from build123d import *

# Parameters (mm, degrees)
SKETCH1_W           = 45.3
SKETCH1_H           = 30
BOSS_EXTRUDE1_DEPTH = 7
SKETCH2_W           = 45.3
SKETCH2_H           = 24.294385672
CUT_EXTRUDE1_DEPTH  = 6
SKETCH5_W           = 12
SKETCH5_H           = 5.5
SKETCH5_W_2         = 10
SKETCH5_H_2         = 7
CUT_EXTRUDE2_DEPTH  = 7


with BuildPart() as part:
    # Sketch1 → Boss-Extrude1 (new body)
    with BuildSketch(Plane.XY):
        with Locations((5.590822785, 11.37721519)):
            Rectangle(SKETCH1_W, SKETCH1_H)
    extrude(amount=BOSS_EXTRUDE1_DEPTH)

    # Sketch2 → Cut-Extrude1 (cut)
    with BuildSketch(Plane.XY.offset(7)):
        with Locations((5.590822785, 8.524408026)):
            Rectangle(SKETCH2_W, SKETCH2_H)
    extrude(amount=-CUT_EXTRUDE1_DEPTH, mode=Mode.SUBTRACT)

    # Sketch5 → Cut-Extrude2 (cut)
    with BuildSketch(Plane(origin=(0, 26.37721519, 0), x_dir=(1, 0, 0), z_dir=(0, 1, 0))):
        with Locations((5.590822785, -2.75)):
            Rectangle(SKETCH5_W, SKETCH5_H)
        with Locations((-12.059177215, -3.5)):
            Rectangle(SKETCH5_W_2, SKETCH5_H_2)
        with Locations((23.240822785, -3.5)):
            Rectangle(SKETCH5_W_2, SKETCH5_H_2)
    extrude(amount=-CUT_EXTRUDE2_DEPTH, mode=Mode.SUBTRACT)


solid = part.part
Read the model definition and answer for the solid it produces. Units are mm, in the model's axes. A direction names the side the tool comes from. Give positions to 0.01 mm unless a question says otherwise; leave off trailing zeros. Write each loop counter-clockwise with the first axis right and the second up, starting at its lowest first coordinate (ties: lowest second). Pieces come first, ordered by that corner, then holes. Notation, with made-up numbers: (-23.5, 86.25) - (31.5, 86.25) arc R24 ccw to (31.5, 104.25) - close; hole circle Ø4 at (17, 47). An arc over 180 degrees is marked (long way). Return JSON: item names as keys, results as strings.
Q1. For faces 1 (the face through (5, 9, 1)), 2 (the face through (5.5, 19.377, 0.5)), 3 (the face through (18.241, 24, 4)), 4 (the face through (6, 24, 5.5)), 5 (the face through (-0.409, 24, 3)), determine the directions among +Z, -Z, +X, -X, +Y, -Y from which every point of the face is accessible in a straight line to the end or side of a thin tool.
Reply:
{"face 1": "+Z, +X, -X, -Y", "face 2": "+Z, -Z, +Y", "face 3": "+Z, -Z, +X, +Y", "face 4": "-Z, +Y, -Y", "face 5": "-Z, +Y"}
Q2. For a pull along X with two mould halves and no side action, classify faces 6 (the face through (11.591, 24, 3)), 7 (the face through (5, 20.672, 6)), 8 (the face through (28.241, 7.7, 0.5)) as released by +X, released by -X, zero draft, split by the parting line, or undercut.
Reply:
{"face 6": "undercut", "face 7": "zero draft", "face 8": "released by +X"}
Q3. Consider line 1 along Z through (x, y) = (2, -1.5); line 2 along X through (y, z) = (25, 3); line 3 along Y through (x, z) = (9.5, 6.75). Determine where each line is inside the solid, lowest interval first. Write a range as [from, to].
Reply:
{"line 1": "[0, 1]", "line 2": "[-7.06, -0.41], [11.59, 18.24]", "line 3": "[20.67, 26.38]"}
Q4. A cutting plane is placed at B-B, the plane x = 4. Determine the outline of the cut face in (y, z), and give its area (3 significant figures).
Reply:
{"outline": "(-3.62, 0) - (19.38, 0) - (19.38, 1) - (-3.62, 1) - close; (20.67, 5.5) - (26.38, 5.5) - (26.38, 7) - (20.67, 7) - close", "area": "31.6 mm²"}
Q5. A cutting plane is placed at A-A, the plane z = 1.75. Determine the outline of the cut face in (x, y), and give its area (3 significant figures).
Reply:
{"outline": "(-7.06, 20.67) - (-0.41, 20.67) - (-0.41, 26.38) - (-7.06, 26.38) - close; (11.59, 20.67) - (18.24, 20.67) - (18.24, 26.38) - (11.59, 26.38) - close", "area": "75.9 mm²"}
Q6. A cutting plane is placed at C-C, the plane x = -6. Determine the outline of the cut face in (y, z), and give its area (3 significant figures).
Reply:
{"outline": "(-3.62, 0) - (26.38, 0) - (26.38, 7) - (20.67, 7) - (20.67, 1) - (-3.62, 1) - close", "area": "64.2 mm²"}
Q7. Given P1, Ø2, axis at x = 18.5, y = 6.5, coming from the +Z side; P2, Ø0.5, axis at x = 23.5, z = 0.5, coming from the +Y side; P3, Ø1.6, axis at y = 23.5, z = 4, coming from the -X side, each flat-ended and moving along its own axis, determine where each tip first touches the part or whether it passes through.
Reply:
{"P1": "z = 1", "P2": "y = 19.38", "P3": "x = -7.06"}
Q8. A cutting plane is placed at D-D, the plane y = 9. Determine the outline of the cut face in (x, z), and give its area (3 significant figures).
Reply:
{"outline": "(-17.06, 0) - (28.24, 0) - (28.24, 1) - (-17.06, 1) - close", "area": "45.3 mm²"}
